For this review, take the finished solid that the model builds, in its own axes (mm). Face numbers are marked on the shaded views. Give positions to 0.01 mm unless a question says otherwise; leave off trailing zeros. Order: outer loops, then holes, each group sorted by start corner. A loop starts at its lowest first (then second) coordinate and runs counter-clockwise, first axis right, second up.
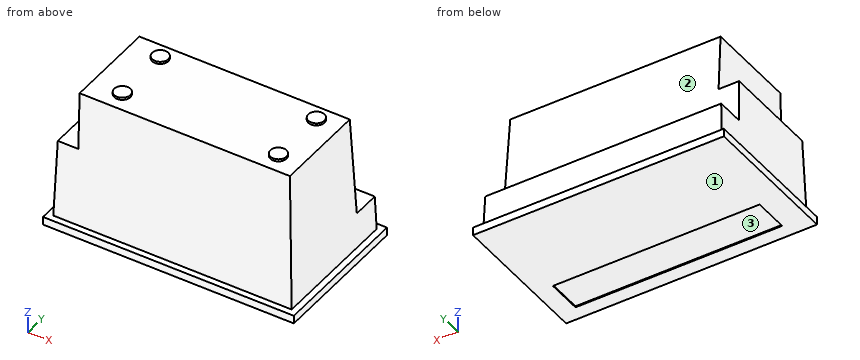
from build123d import *

# Parameters (mm, degrees)
SKETCH_1_W               = 103
SKETCH_1_H               = 57
EXTRUDE_1_DEPTH          = 59
EXTRUDE_1_TAPER          = 2
SKETCH_2_W               = 39.54031551
SKETCH_2_H               = 84.548972525
CUT_EXTRUDE_1_DEPTH      = 25
SKETCH_3_R               = 3.5
EXTRUDE_2_DEPTH          = 1
SKETCH_4_W               = 108.4
SKETCH_4_H               = 62.4
EXTRUDE_3_DEPTH          = 3.5
CUT_EXTRUDE_2_DEPTH      = 87.666487179
CUT_EXTRUDE_2_DEPTH_BACK = 87.666487179
SKETCH_6_W               = 89.310356146
SKETCH_6_H               = 15.122271459
CUT_EXTRUDE_3_DEPTH      = 0.5


with BuildPart() as part:
    # 草图1 → 拉伸1 (new body)
    with BuildSketch(Plane.XY):
        Rectangle(SKETCH_1_W, SKETCH_1_H)
    extrude(amount=EXTRUDE_1_DEPTH, taper=EXTRUDE_1_TAPER)

    # 草图2 → 切除-拉伸1 (cut)
    with BuildSketch(Plane.XY.offset(59)):
        with Locations((-61.209832355, 4.206416544)):
            Rectangle(SKETCH_2_W, SKETCH_2_H)
    extrude(amount=-CUT_EXTRUDE_1_DEPTH, mode=Mode.SUBTRACT)

    # 草图3 → 拉伸2 (add)
    with BuildSketch(Plane.XY.offset(59)):
        with Locations((-28.146233383, 6.977331271)):
            Circle(SKETCH_3_R)
        with Locations((39.303298868, 6.977331271)):
            Circle(SKETCH_3_R)
        with Locations((-28.146233383, -18.443352833)):
            Circle(SKETCH_3_R)
        with Locations((39.303298868, -18.443352833)):
            Circle(SKETCH_3_R)
    extrude(amount=EXTRUDE_2_DEPTH)

    # 草图4 → 拉伸3 (add)
    with BuildSketch(Plane(origin=(0, 0, 0), x_dir=(-1, 0, 0), z_dir=(0, 0, -1))):
        Rectangle(SKETCH_4_W, SKETCH_4_H)
    extrude(amount=EXTRUDE_3_DEPTH)

    # 草图5 → 切除-拉伸2 (cut, two sides: drawn at the far end of the back side and taken through both)
    with BuildSketch(Plane(origin=(0, 0, 0), x_dir=(0, 0, -1), z_dir=(1, 0, 0)).offset(-CUT_EXTRUDE_2_DEPTH_BACK)):
        Polygon((-59, 13.626611521), (-15, 15.976188458), (-15, 27.976188458), (-59, 29.657919194), align=None)
    extrude(amount=CUT_EXTRUDE_2_DEPTH + CUT_EXTRUDE_2_DEPTH_BACK, mode=Mode.SUBTRACT)

    # 草图6 → 切除-拉伸3 (cut)
    with BuildSketch(Plane(origin=(0, 0, -3.5), x_dir=(-1, 0, 0), z_dir=(0, 0, -1))):
        with Locations((-1.512227146, -17.435089447)):
            Rectangle(SKETCH_6_W, SKETCH_6_H)
    extrude(amount=-CUT_EXTRUDE_3_DEPTH, mode=Mode.SUBTRACT)


solid = part.part
1) Clearance check with flat-ended pins moving along their axes: pin 1 (6 mm diameter, centred on x = -18, z = 25, fed in from +Y); pin 2 (12 mm diameter, centred on y = -3, z = 45.5, fed in from +X); pin 3 (2 mm diameter, centred on y = 10, z = 23.5, fed in from +X). State where each tip first meets the part, or that it passes through.
Answer sheet:
pin 1: stops at y = 15.6
pin 2: stops at x = 50.12
pin 3: stops at x = 50.71
2) We need section C-C on z = 51.5. Give the boundary of the cut face in (x, y), then the cut area to 3 significant figures.
Answer sheet:
outline: (-41.44, -26.7) - (49.7, -26.7) - (49.7, 14.03) - (-41.44, 14.03) - close
area: 3,710 mm2
3) We need section B-B on y = -6. Give the boundary of the cut face in (x, z), then the cut area to 3 significant figures.
Answer sheet:
outline: (-54.2, -3.5) - (54.2, -3.5) - (54.2, 0) - (51.5, 0) - (49.44, 59) - (-41.44, 59) - (-41.44, 34) - (-50.31, 34) - (-51.5, 0) - (-54.2, 0) - close
area: 6,120 mm2
4) To check wall thickness, follow line 1 (Z direction, x = 19, y = -8); line 2 (Z direction, x = -48.5, y = -21.5); line 3 (X direction, y = -1, z = 40.5). State the ranges of each line that lie inside material, in increasing order.
Answer sheet:
line 1: z = -3.5 to 59
line 2: z = -3.5 to 34
line 3: x = -41.44 to 50.09
5) We need section D-D on x = 38.5. Give the boundary of the cut face in (y, z), then the cut area to 3 significant figures.
Answer sheet:
outline: (-31.2, -3.5) - (-25, -3.5) - (-25, -3) - (-9.87, -3) - (-9.87, -3.5) - (31.2, -3.5) - (31.2, 0) - (28.5, 0) - (27.98, 15) - (15.98, 15) - (13.63, 59) - (10.38, 59) - (10.38, 60) - (3.57, 60) - (3.57, 59) - (-15.04, 59) - (-15.04, 60) - (-21.85, 60) - (-21.85, 59) - (-26.44, 59) - (-28.5, 0) - (-31.2, 0) - close
area: 2,920 mm2
6) Draft analysis for pull direction Y (two halves, no side actions). For the marked faces 1, 2 and 3, state which applies: +Y half, -Y half, draft (parallel to the pull), parting line (faces both ways), or undercut.
Answer sheet:
face 1: draft
face 2: +Y half
face 3: undercut
7) We need section A-A on x = 12.5. Give the boundary of the cut face in (y, z), then the cut area to 3 significant figures.
Answer sheet:
outline: (-31.2, -3.5) - (-25, -3.5) - (-25, -3) - (-9.87, -3) - (-9.87, -3.5) - (31.2, -3.5) - (31.2, 0) - (28.5, 0) - (27.98, 15) - (15.98, 15) - (13.63, 59) - (-26.44, 59) - (-28.5, 0) - (-31.2, 0) - close
area: 2,910 mm2
